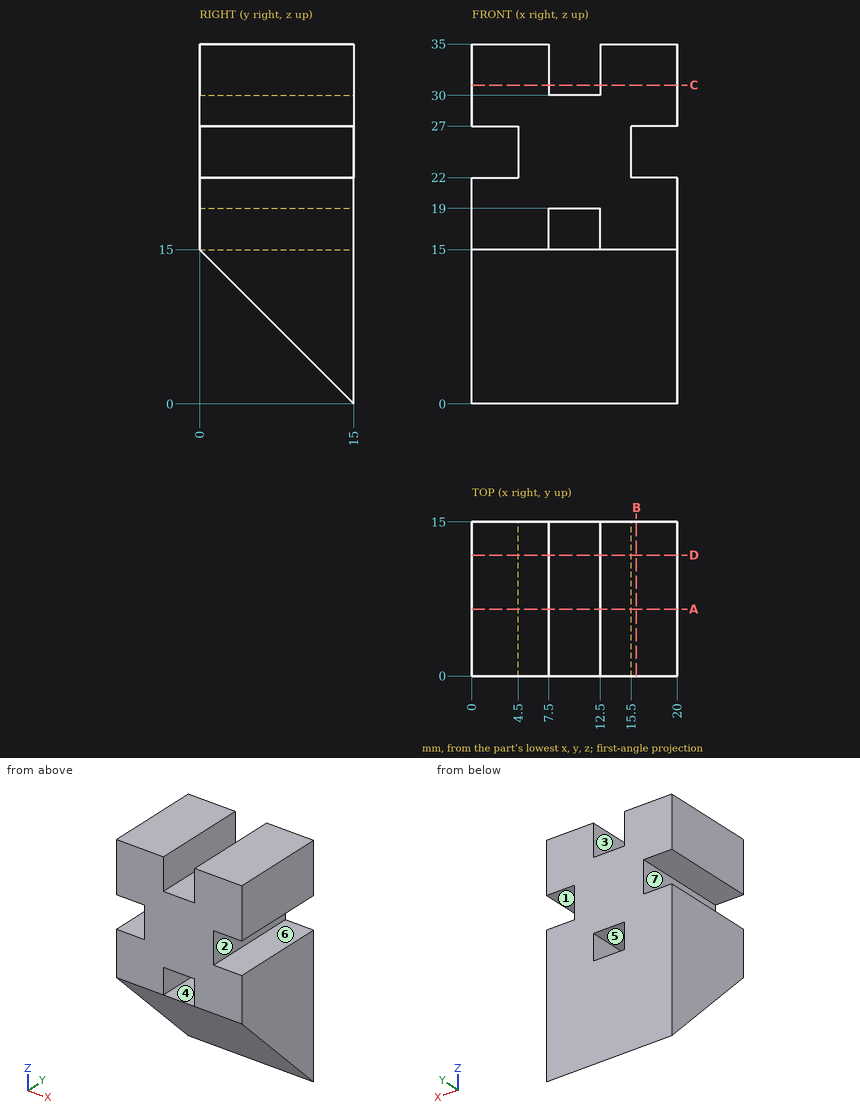
Answer from the drawing. Dimensions are ordinates in mm from the lowest x, y and z of the part. A direction names the side the tool comes from. Round coordinates to 2 decimals unless told otherwise and drop trailing zeros. Write each loop counter-clockwise with the first axis right and the second up, starting at its lowest first coordinate (ties: lowest second). Pieces come first, ordered by that corner, then holes. Notation, with made-up numbers: M -16,58 L 26,58 A24 ccw 26,97 Z; hole C 88.25,0 d8. An arc over 180 degrees is marked long. Write each question's results on one line, items separated by ' | '. Start each with the question number.
Item 1: Flat-ended cylindrical pins translate along their axes: pin 1 Ø3.5 at (x, y) = (16.5, 6.5) entering from -Z; pin 2 Ø2 at (x, y) = (3.5, 8) entering from -Z; pin 3 Ø6 at (x, y) = (10.5, 5) entering from -Z. Find the tip coordinate at first contact, or state that the pin passes through.
Item 2: For the marked faces 5, 6 and 7, determine the directions among +Z, -Z, +X, -X, +Y, -Y from which every point of the face is accessible in a straight line to the end or side of a thin tool.
Item 3: For a pull along X with two mould halves and no side action, classify the marked faces 1, 2, 3 and 4 as pulls with the +X half, pulls with the -X half, needs draft (parallel to the pull), parting line crosses it, or undercut.
Item 4: A cutting plane is placed at A-A on y = 6.5. Write down the section's boundary in (x, z), and give its area (3 significant figures).
Item 5: A cutting plane is placed at C-C on z = 31. Write down the section's boundary in (x, y), and give its area (3 significant figures).
Item 6: A cutting plane is placed at D-D on y = 11.75. Write down the section's boundary in (x, z).
Item 7: Straight lines are drawn through the part: L1, parallel to X at y = 2.5, z = 32.5; L2, parallel to X at y = 11, z = 24.5; L3, parallel to Z at x = 12, y = 2.5. For each, find the intervals that lie inside material, in ascending order. Write a range as [from, to].
Item 8: A cutting plane is placed at B-B on x = 16. Write down the section's boundary in (y, z), and give its area (4 significant figures).
Check sheet entries:
1) pin 1: z = 6.75 | pin 2: z = 6 | pin 3: z = 7
2) face 5: +Y, -Y | face 6: +X, +Y, -Y | face 7: -X, +Y, -Y
3) face 1: needs draft | face 2: pulls with the +X half | face 3: undercut | face 4: undercut
4) outline: M 0,8.5 L 20,8.5 L 20,22 L 15.5,22 L 15.5,27 L 20,27 L 20,35 L 12.5,35 L 12.5,30 L 7.5,30 L 7.5,35 L 0,35 L 0,27 L 4.5,27 L 4.5,22 L 0,22 Z; hole M 7.5,15 L 12.5,15 L 12.5,19 L 7.5,19 Z | area: 440 mm²
5) outline: M 0,0 L 7.5,0 L 7.5,15 L 0,15 Z; M 12.5,0 L 20,0 L 20,15 L 12.5,15 Z | area: 225 mm²
6) outline: M 0,3.25 L 20,3.25 L 20,22 L 15.5,22 L 15.5,27 L 20,27 L 20,35 L 12.5,35 L 12.5,30 L 7.5,30 L 7.5,35 L 0,35 L 0,27 L 4.5,27 L 4.5,22 L 0,22 Z; hole M 7.5,15 L 12.5,15 L 12.5,19 L 7.5,19 Z
7) L1: [0, 7.5], [12.5, 20] | L2: [4.5, 15.5] | L3: [12.5, 15], [19, 30]
8) outline: M 0,15 L 15,0 L 15,22 L 0,22 Z; M 0,27 L 15,27 L 15,35 L 0,35 Z | area: 337.5 mm²
